Part model, mm, in its own coordinate system. A direction names the side the tool comes from. Coordinates: 2 decimals unless noted, no trailing zeros. Order: outer loops, then holes, each group sorted by start corner. A loop starts at its lowest first (then second) coordinate and runs counter-clockwise, first axis right, second up.
1) Wall check: L1, parallel to Z at x = 6, y = -3.75 (3 decimals); L2, parallel to Z at x = 18, y = -4.45 (3 decimals); L3, parallel to Z at x = 8, y = 4. Give the ranges that are in metal, low to high.
2) Pin check, flat tips, straight feed: pin 1 Ø5 at (x, y) = (15.5, -10) entering from +Z; pin 2 Ø3.5 at (x, y) = (10, 7) entering from +Z; pin 3 Ø2.5 at (x, y) = (-6.5, -2) entering from -Z; pin 4 Ø2.5 at (x, z) = (5.5, 18.5) entering from -Y. Stop position of each tip, or through.
3) Tool access for faces 4 (the flat face through (6, -9, 12)), 5 (the flat face through (6, 5, 9)), 6 (the flat face through (9, 8, 8)), 7 (the flat face through (18, -9, 3)): list every direction of +Z, -Z, +X, -X, +Y, -Y with a clear straight run to the whole face (end or side of a thin tool).
4) Cut at D-D (x = -0.5). List the corners of the cut face in (y, z).
5) Cut at B-B (y = -5.5). List the corners of the cut face in (x, z) (3 decimals), and give its area (3 significant figures).
6) Cut at A-A (x = 18). List the corners of the cut face in (y, z) (3 decimals).
7) Cut at C-C (x = 10). List the corners of the cut face in (y, z), and give its area (3 significant figures).
8) Mould opens along Z. For faces 1 (the flat face through (-6, -9, 3)), 2 (the flat face through (18, -1, 10.35)), 3 (the flat face through (-12, -5, 5)) say: +Z half, -Z half, draft (parallel to the pull), parting line (faces both ways), or undercut.
Autodesk Inventor part; units mm, degrees
ref_plane "YZ Plane" through (0, 0, 0) normal (1, 0, 0) x (0, 1, 0)
ref_plane "XZ Plane" through (0, 0, 0) normal (0, 1, 0) x (-1, 0, 0)
ref_plane "XY Plane" through (0, 0, 0) normal (0, 0, 1) x (1, 0, 0)
sketch "Sketch1" plane through (0, 0, 0) normal (0, 0, 1) x (1, 0, 0)
  line L0 (0, 0) -> (12, 0)
  line L1 (12, 0) -> (12, 12)
  line L2 (12, 12) -> (0, 12)
  line L3 (0, 12) -> (0, 0)
  line L4 (12, 0) -> (0, 0)
  line L5 (0, 0) -> (0, -12)
  line L6 (0, -12) -> (12, -12)
  line L7 (12, -12) -> (12, 0)
  line L8 (12, 0) -> (24, 0)
  line L9 (24, 0) -> (24, -12)
  line L10 (24, -12) -> (12, -12)
  line L11 (12, -12) -> (12, 0)
  line L12 (0, -12) -> (-12, -12)
  line L13 (-12, -12) -> (-12, 0)
  line L14 (-12, 0) -> (0, 0)
  line L15 (0, 0) -> (0, -12)
  line L16 (0, -12) -> (12, -12)
  line L17 (12, -12) -> (12, -24)
  line L18 (12, -24) -> (0, -24)
  line L19 (0, -24) -> (0, -12)
  dimension "d0" = 12
  dimension "d1" = 12
  dimension "d2" = 12
  dimension "d3" = 12
  dimension "d4" = 12
  dimension "d5" = 12
  dimension "d6" = 12
  dimension "d7" = 12
  dimension "d8" = 12
  dimension "d9" = 12
extrude "Extrusion1" add sketch "Sketch1" along normal blind 3
sketch "Sketch2" plane through (0, 0, 3) normal (0, 0, 1) x (1, 0, 0)
  line L0 (-12, 0) -> (-12, -12)
  line L1 (-12, -12) -> (-12, -6)
  line L2 (-12, -6) -> (0, -6)
  line L3 (-12, -12) -> (0, -12)
  line L4 (0, -6) -> (0, -12)
  line L5 (0, -12) -> (-12, -12)
  line L6 (12, -24) -> (12, -12)
  line L7 (12, -12) -> (12, -6)
  line L8 (12, -6) -> (24, -6)
  line L9 (24, -12) -> (24, 0)
  line L10 (12, -12) -> (24, -12)
  line L11 (24, -6) -> (24, -12)
  line L12 (24, -12) -> (12, -12)
  line L13 (0, 0) -> (0, -6)
  line L14 (12, 0) -> (12, 12)
  line L15 (0, 0) -> (12, 0)
  line L16 (12, 0) -> (12, -6)
  line L17 (12, -12) -> (0, -12)
  line L18 (0, 12) -> (0, 0)
  line L19 (0, 0) -> (0, 12)
  line L20 (0, 12) -> (6, 12)
  line L21 (12, 12) -> (0, 12)
  line L22 (6, 12) -> (6, 0)
  line L23 (6, 0) -> (0, 0)
  line L24 (0, -12) -> (0, -24)
  line L25 (0, -12) -> (0, -24)
  line L26 (0, -24) -> (6, -24)
  line L27 (0, -24) -> (12, -24)
  line L28 (6, -24) -> (6, -12)
  line L29 (6, -12) -> (0, -12)
  dimension "d12" = 6
  dimension "d13" = 12
extrude "Extrusion2" add sketch "Sketch2" along normal blind 9 contours L2 L4 L3 L0 | L13 L15 L16 L7 L17 L4 | L17 L28 L26 L24 | L18 L20 L22 L15 | L7 L8 L9 L10
sketch "Sketch3" plane through (0, 0, 12) normal (0, 0, 1) x (1, 0, 0)
  line L0 (0, -6) -> (12, -6)
  line L1 (12, -12) -> (6, -12)
  line L2 (12, -6) -> (12, -12)
  line L3 (0, -12) -> (0, -24)
  line L4 (12, -12) -> (0, -12)
  line L5 (0, -12) -> (0, -6)
  point P0 (0, 0)
extrude "Extrusion3" add sketch "Sketch3" along normal blind 9
sketch "Sketch4" plane through (6, -12, 3) normal (0, -1, 0) x (1, 0, 0)
  point P0 (-6, -3)
sketch "Sketch5" plane through (-12, -6, 3) normal (0, 1, 0) x (1, 0, 0)
  circle A0 centre (6, -4.5) radius 1.725
  line L0 (0, 0) -> (0, -9)
  line L1 (12, -9) -> (0, -9)
  circle A1 centre (18, -13.5) radius 1.725
  line L2 (24, -18) -> (12, -18)
  line L3 (24, -9) -> (24, -18)
  circle A2 centre (30, -4.5) radius 1.725
  line L4 (36, 0) -> (36, -9)
  line L5 (36, -9) -> (24, -9)
  point P0 (12, 3)
  dimension "d19" = 3.45
  dimension "d20" = 6
  dimension "d21" = 4.5
  dimension "d22" = 3.45
  dimension "d23" = 4.5
  dimension "d24" = 6
  dimension "d25" = 3.45
  dimension "d26" = 6
  dimension "d27" = 4.5
extrude "Extrusion4" cut sketch "Sketch5" against normal blind 3
sketch "Sketch6" plane through (6, -12, 3) normal (0, -1, 0) x (1, 0, 0)
  circle A0 centre (-12, 4.5) radius 1.725
  line L0 (-10.3546, 7.35) -> (-8.7091, 4.5)
  line L1 (-8.7091, 4.5) -> (-10.3546, 1.65)
  line L2 (-10.3546, 1.65) -> (-13.6454, 1.65)
  line L3 (-13.6454, 1.65) -> (-15.2909, 4.5)
  line L4 (-15.2909, 4.5) -> (-13.6454, 7.35)
  line L5 (-13.6454, 7.35) -> (-10.3546, 7.35)
  circle A1 centre (12, 4.5) radius 1.725
  line L6 (13.6454, 7.35) -> (15.2909, 4.5)
  line L7 (15.2909, 4.5) -> (13.6454, 1.65)
  line L8 (13.6454, 1.65) -> (10.3546, 1.65)
  line L9 (10.3546, 1.65) -> (8.7091, 4.5)
  line L10 (8.7091, 4.5) -> (10.3546, 7.35)
  line L11 (10.3546, 7.35) -> (13.6454, 7.35)
  circle A2 centre (0, 13.5) radius 1.725
  line L12 (1.6454, 16.35) -> (3.2909, 13.5)
  line L13 (3.2909, 13.5) -> (1.6454, 10.65)
  line L14 (1.6454, 10.65) -> (-1.6454, 10.65)
  line L15 (-1.6454, 10.65) -> (-3.2909, 13.5)
  line L16 (-3.2909, 13.5) -> (-1.6454, 16.35)
  line L17 (-1.6454, 16.35) -> (1.6454, 16.35)
  point P0 (-6, -3)
  dimension "d30" = 2.85
  dimension "d31" = 2.85
  dimension "d32" = 2.85
extrude "Extrusion5" cut sketch "Sketch6" against normal blind 3 contours A0 | L0 L1 L2 L3 L4 L5 | A1 | L6 L7 L8 L9 L10 L11 | A2 | L12 L13 L14 L15 L16 L17
sketch "Sketch7" plane through (6, 0, 3) normal (1, 0, 0) x (0, 0, -1)
  circle A0 centre (-4.5, 6) radius 1.725
  circle A1 centre (-4.5, -18) radius 1.725
  line L0 (-9, 0) -> (-9, 12)
  line L1 (-9, -24) -> (-9, -12)
  line L2 (0, -24) -> (-9, -24)
  line L3 (0, 12) -> (-9, 12)
  point P0 (3, 0)
  dimension "d35" = 3.45
  dimension "d36" = 3.45
  dimension "d37" = 4.5
  dimension "d38" = 4.5
  dimension "d39" = 6
  dimension "d40" = 6
extrude "Extrusion6" cut sketch "Sketch7" against normal blind 3
sketch "Sketch8" plane through (0, -6, 3) normal (-1, 0, 0) x (0, 0, 1)
  circle A0 centre (4.5, 12) radius 1.725
  line L0 (1.65, 13.6454) -> (4.5, 15.2909)
  line L1 (4.5, 15.2909) -> (7.35, 13.6454)
  line L2 (7.35, 13.6454) -> (7.35, 10.3546)
  line L3 (7.35, 10.3546) -> (4.5, 8.7091)
  line L4 (4.5, 8.7091) -> (1.65, 10.3546)
  line L5 (1.65, 10.3546) -> (1.65, 13.6454)
  circle A1 centre (4.5, -12) radius 1.725
  line L6 (1.65, -10.3546) -> (4.5, -8.7091)
  line L7 (4.5, -8.7091) -> (7.35, -10.3546)
  line L8 (7.35, -10.3546) -> (7.35, -13.6454)
  line L9 (7.35, -13.6454) -> (4.5, -15.2909)
  line L10 (4.5, -15.2909) -> (1.65, -13.6454)
  line L11 (1.65, -13.6454) -> (1.65, -10.3546)
  point P0 (-3, 6)
  dimension "d43" = 2.85
  dimension "d44" = 2.85
extrude "Extrusion7" cut sketch "Sketch8" against normal blind 3 contours A0 | L0 L1 L2 L3 L4 L5 | A1 | L6 L7 L8 L9 L10 L11
sketch "Sketch9" plane through (0, 0, 0) normal (0, 0, -1) x (-1, 0, 0)
  line L0 (-24, -12) -> (-24, 0)
  line L1 (-12, -12) -> (-12, -6)
  line L2 (-24, 0) -> (-12, 0)
  line L3 (-12, 0) -> (-12, -12)
  line L4 (-12, -12) -> (-24, -12)
  line L5 (-24, -12) -> (-24, 0)
  line L6 (-12, -12) -> (0, -12)
  line L7 (0, -12) -> (0, -24)
  line L8 (0, -24) -> (-12, -24)
  line L9 (-12, -24) -> (-12, -12)
  point P0 (0, 0)
extrude "Extrusion8" cut sketch "Sketch9" against normal through all
sketch "Sketch10" plane through (0, 12, 12) normal (0, 1, 0) x (1, 0, 0)
  line L0 (6, 0) -> (0, 0)
  line L1 (12, 9) -> (6, 9)
  line L2 (0, 0) -> (6, 0)
  line L3 (6, 0) -> (6, 9)
  line L4 (6, 9) -> (0, 9)
  line L5 (0, 9) -> (0, 0)
  point P0 (0, 12)
extrude "Extrusion9" cut sketch "Sketch10" against normal blind 12
sketch "Sketch11" plane through (0, 0, 3) normal (0, 1, 0) x (1, 0, 0)
  line L0 (12, 0) -> (12, -9)
  line L1 (12, 0) -> (0, 0)
  line L2 (12, -9) -> (6, -9)
  line L3 (6, -9) -> (6, 0)
  line L4 (6, 0) -> (12, 0)
  line L5 (12, 0) -> (12, -9)
  point P0 (0, 3)
extrude "Extrusion10" add sketch "Sketch11" along normal blind 12
sketch "Sketch12" plane through (6, 0, 3) normal (-1, 0, 0) x (0, 0, 1)
  circle A0 centre (4.5, 6) radius 1.575
  line L0 (9, 0) -> (9, 12)
  line L1 (0, 12) -> (9, 12)
  point P0 (-3, 0)
  dimension "d54" = 3.15
  dimension "d55" = 4.5
  dimension "d56" = 6
extrude "Extrusion11" cut sketch "Sketch12" against normal blind 3
sketch "Sketch13" plane through (12, -6, 12) normal (1, 0, 0) x (0, 0, -1)
  circle A0 centre (4.5, 12) radius 1.575
  line L0 (1.65, 13.6454) -> (4.5, 15.2909)
  line L1 (4.5, 15.2909) -> (7.35, 13.6454)
  line L2 (7.35, 13.6454) -> (7.35, 10.3546)
  line L3 (7.35, 10.3546) -> (4.5, 8.7091)
  line L4 (4.5, 8.7091) -> (1.65, 10.3546)
  line L5 (1.65, 10.3546) -> (1.65, 13.6454)
  point P0 (12, 6)
  dimension "d59" = 5.7
extrude "Extrusion12" cut sketch "Sketch13" against normal blind 3 contours A0 | L0 L1 L2 L3 L4 L5
sketch "Sketch14" plane through (0, -6, 3) normal (-1, 0, 0) x (0, 0, 1)
  line L0 (9, 6) -> (0, 6)
  line L1 (0, 6) -> (0, 0)
  line L2 (9, 6) -> (0, 6)
  line L3 (0, 6) -> (0, 0)
  line L4 (0, 0) -> (9, 0)
  line L5 (9, 0) -> (9, 6)
  point P0 (-3, 6)
extrude "Extrusion13" add sketch "Sketch14" along normal blind 12
sketch "Sketch15" plane through (-12, -12, 0) normal (-1, 0, 0) x (0, 0, 1)
  line L0 (12, 0) -> (12, 6)
  line L1 (12, 0) -> (3, 0)
  line L2 (3, 0) -> (3, 6)
  line L3 (3, 6) -> (12, 6)
  line L4 (12, 6) -> (12, 0)
  point P0 (0, 12)
  dimension "d64" = 9
  dimension "d65" = 6
extrude "Extrusion14" cut sketch "Sketch15" against normal blind 12
sketch "Sketch16" plane through (-12, -6, 12) normal (0, -1, 0) x (1, 0, 0)
  circle A0 centre (6, -4.5) radius 1.725
  line L0 (0, -9) -> (0, 0)
  line L1 (0, 0) -> (12, 0)
  point P0 (12, -12)
  dimension "d68" = 3.45
  dimension "d69" = 6
  dimension "d70" = 4.5
extrude "Extrusion15" cut sketch "Sketch16" against normal blind 3
sketch "Sketch17" plane through (-12, 0, 0) normal (0, 1, 0) x (1, 0, 0)
  circle A0 centre (6, -7.5) radius 1.725
  line L0 (4.3546, -10.35) -> (2.7091, -7.5)
  line L1 (2.7091, -7.5) -> (4.3546, -4.65)
  line L2 (4.3546, -4.65) -> (7.6454, -4.65)
  line L3 (7.6454, -4.65) -> (9.2909, -7.5)
  line L4 (9.2909, -7.5) -> (7.6454, -10.35)
  line L5 (7.6454, -10.35) -> (4.3546, -10.35)
  point P0 (12, 0)
  dimension "d73" = 5.7
extrude "Extrusion16" cut sketch "Sketch17" against normal blind 3 contours A0 | L0 L1 L2 L3 L4 L5
sketch "Sketch18" plane through (0, 0, 12) normal (0, 0, 1) x (1, 0, 0)
  line L0 (12, -6) -> (12, 12)
  line L1 (0, 0) -> (12, 0)
  line L2 (12, 0) -> (12, -6)
  line L3 (12, -6) -> (0, -6)
  line L4 (0, -6) -> (0, 0)
extrude "Extrusion17" add sketch "Sketch18" along normal blind 9
sketch "Sketch19" plane through (0, 0, 21) normal (0, 0, 1) x (1, 0, 0)
  line L0 (0, -12) -> (12, -12)
  line L1 (12, -12) -> (12, 0)
  line L2 (0, -12) -> (12, -12)
  line L3 (12, -12) -> (12, -6)
  line L4 (12, -6) -> (0, -6)
  line L5 (0, -6) -> (0, -12)
  point P0 (0, 0)
extrude "Extrusion18" cut sketch "Sketch19" against normal blind 9
sketch "Sketch20" plane through (0, -6, 21) normal (0, -1, 0) x (1, 0, 0)
  circle A0 centre (6, -4.5) radius 1.725
  line L0 (0, 0) -> (12, 0)
  line L1 (0, -9) -> (0, 0)
  point P0 (0, -21)
  dimension "d80" = 3.45
  dimension "d81" = 4.5
  dimension "d82" = 6
extrude "Extrusion19" cut sketch "Sketch20" against normal blind 3
sketch "Sketch21" plane through (-12, 0, 0) normal (0, 1, 0) x (1, 0, 0)
  circle A0 centre (18, -16.5) radius 1.725
  line L0 (16.3546, -19.35) -> (14.7091, -16.5)
  line L1 (14.7091, -16.5) -> (16.3546, -13.65)
  line L2 (16.3546, -13.65) -> (19.6454, -13.65)
  line L3 (19.6454, -13.65) -> (21.2909, -16.5)
  line L4 (21.2909, -16.5) -> (19.6454, -19.35)
  line L5 (19.6454, -19.35) -> (16.3546, -19.35)
  point P0 (12, 0)
  dimension "d85" = 5.7
extrude "Extrusion20" cut sketch "Sketch21" against normal blind 3 contours A0 | L0 L1 L2 L3 L4 L5
sketch "Sketch22" plane through (12, -12, 0) normal (1, 0, 0) x (0, 0, -1)
  line L0 (-12, 6) -> (-12, 12)
  line L1 (0, 24) -> (0, 12)
  line L2 (-12, 6) -> (-3, 6)
  line L3 (0, 0) -> (0, 12)
  line L4 (0, 12) -> (-12, 12)
  line L5 (-12, 12) -> (-12, 6)
  line L6 (0, 0) -> (-12, 0)
  line L7 (-3, 6) -> (-12, 6)
  line L8 (0, 0) -> (-3, 0)
  line L9 (-3, 0) -> (-3, 6)
  line L10 (0, 12) -> (0, 0)
extrude "Extrusion21" add sketch "Sketch22" along normal blind 12
sketch "Sketch23" plane through (12, -6, 3) normal (0, -1, 0) x (1, 0, 0)
  circle A0 centre (6, 4.5) radius 1.725
  line L0 (0, 9) -> (12, 9)
  line L1 (12, 9) -> (12, 0)
  point P0 (-12, -3)
  dimension "d91" = 3.45
  dimension "d92" = 4.5
  dimension "d93" = 6
extrude "Extrusion22" cut sketch "Sketch23" against normal blind 3
sketch "Sketch24" plane through (12, 0, 12) normal (0, 1, 0) x (1, 0, 0)
  circle A0 centre (6, 4.5) radius 1.725
  line L0 (4.3546, 1.65) -> (2.7091, 4.5)
  line L1 (2.7091, 4.5) -> (4.3546, 7.35)
  line L2 (4.3546, 7.35) -> (7.6454, 7.35)
  line L3 (7.6454, 7.35) -> (9.2909, 4.5)
  line L4 (9.2909, 4.5) -> (7.6454, 1.65)
  line L5 (7.6454, 1.65) -> (4.3546, 1.65)
  point P0 (-12, 12)
  dimension "d96" = 5.7
extrude "Extrusion23" cut sketch "Sketch24" against normal blind 3 contours A0 | L0 L1 L2 L3 L4 L5
fillet "Fillet4" radius 1.5 5 edges at (6, -12, 0) (-6, 0, 0) (0, 6, 0) (12, 6, 0) (18, 0, 0)
properties part number "topthreewayESW"
Geometry check:
1. L1: z = 0 to 14.775, 18.225 to 21
1. L2: z = 0 to 5.775, 9.225 to 12
1. L3: z = 0 to 12
2. pin 1: stops at z = 3
2. pin 2: stops at z = 12
2. pin 3: stops at z = 0
2. pin 4: stops at y = -6
3. face 4: +Z, +X, -X, -Y
3. face 5: +Z, -X, +Y
3. face 6: +X
3. face 7: +Z, +X, -Y
4. outline: (-12, 1.5) arc R1.5 ccw to (-10.5, 0) - (-1.5, 0) arc R1.5 ccw to (0, 1.5) - (0, 12) - (-6, 12) - (-6, 3) - (-12, 3) - close
5. outline: (-12, 0) - (24, 0) - (24, 12) - (12, 12) - (12, 21) - (0, 21) - (0, 12) - (-12, 12) - close; hole circle Ø3.45 at (-6, 7.5); hole circle Ø3.45 at (6, 16.5); hole circle Ø3.45 at (18, 7.5)
5. area: 512 mm2
6. outline: (-12, 1.5) arc R1.5 ccw to (-10.5, 0) - (-1.5, 0) arc R1.5 ccw to (0, 1.5) - (0, 4.65) - (-3, 4.65) - (-3, 5.775) - (-6, 5.775) - (-6, 3) - (-12, 3) - close; (-6, 9.225) - (-3, 9.225) - (-3, 10.35) - (0, 10.35) - (0, 12) - (-6, 12) - close
7. outline: (-12, 1.5) arc R1.5 ccw to (-10.5, 0) - (12, 0) - (12, 12) - (0, 12) - (0, 21) - (-6, 21) - (-6, 12) - (-12, 12) - close; hole (2.71, 7.5) - (4.35, 4.65) - (7.65, 4.65) - (9.29, 7.5) - (7.65, 10.35) - (4.35, 10.35) - close
7. area: 313 mm2
8. face 1: +Z half
8. face 2: undercut
8. face 3: draft
